The model under review builds one solid part; all positions refer to its coordinate system, in mm. A direction names the side the tool comes from. Round coordinates to 2 decimals unless told otherwise and drop trailing zeros. Write each loop counter-clockwise with the first axis right and the second up, starting at its lowest first coordinate (ties: lowest second). Pieces come first, ordered by that corner, then holes. Notation, with made-up numbers: (8.25, 23) - (20.25, 23) arc R25 cw to (20.25, 35) - close; hole circle Ø4 at (57, 6). An arc over 180 degrees is marked (long way). Return JSON: item names as keys, results as strings.
from build123d import *

# Parameters (mm, degrees)
SKETCH_2_W          = 94.5
SKETCH_2_H          = 98.5
EXTRUDE_1_DEPTH     = 35.7
SHELL_1_T           = -1
SKETCH_5_W          = 35.076830759
SKETCH_5_H          = 6.451639633
CUT_EXTRUDE_1_DEPTH = 2
SKETCH_3_R          = 1.75
CUT_EXTRUDE_2_DEPTH = 2


with BuildPart() as part:
    # 草图2 → 凸台-拉伸1 (new body)
    with BuildSketch(Plane.XY):
        with Locations((47.25, 49.25)):
            Rectangle(SKETCH_2_W, SKETCH_2_H)
    extrude(amount=EXTRUDE_1_DEPTH)

    # 抽壳1
    shell_1_openings = [part.faces().sort_by_distance(p)[0] for p in [
        (47.25, 49.25, 35.7),
    ]]
    offset(amount=SHELL_1_T, openings=shell_1_openings, kind=Kind.INTERSECTION)

    # 草图5 → 切除-拉伸1 (cut, through all)
    with BuildSketch(Plane(origin=(0, 1, 0), x_dir=(1, 0, 0), z_dir=(0, 1, 0))):
        with Locations((47.144981411, -7.555579656)):
            Rectangle(SKETCH_5_W, SKETCH_5_H)
    extrude(amount=-CUT_EXTRUDE_1_DEPTH, mode=Mode.SUBTRACT)

    # 草图3 → 切除-拉伸2 (cut, through all)
    with BuildSketch(Plane.XY.offset(1)):
        with Locations((4.75, 49.25)):
            Circle(SKETCH_3_R)
        with Locations((17.1979618, 19.1979618)):
            Circle(SKETCH_3_R)
        with Locations((47.25, 6.75)):
            Circle(SKETCH_3_R)
        with Locations((77.302038201, 19.1979618)):
            Circle(SKETCH_3_R)
        with Locations((89.75, 49.25)):
            Circle(SKETCH_3_R)
        with Locations((77.302038201, 79.3020382)):
            Circle(SKETCH_3_R)
        with Locations((47.25, 91.75)):
            Circle(SKETCH_3_R)
        with Locations((17.1979618, 79.3020382)):
            Circle(SKETCH_3_R)
    extrude(amount=-CUT_EXTRUDE_2_DEPTH, mode=Mode.SUBTRACT)


solid = part.part
(1) Wall thickness on line 1 (Y direction, x = 47.25, z = 0.7); line 2 (Y direction, x = 58, z = 29); line 3 (X direction, y = 38, z = 26): over which ranges is each line inside the solid? List them lowest first.
Filled in:
{"line 1": "y = 0 to 5, 8.5 to 90, 93.5 to 98.5", "line 2": "y = 0 to 1, 97.5 to 98.5", "line 3": "x = 0 to 1, 93.5 to 94.5"}
(2) Mouldability with a two-part tool opening along Y and no side actions: class faces 3 (the flat face through (47, 98.5, 18)), 4 (the cylindrical face through (48.867, 6.08, 0.507)), 5 (the flat face through (47, 97.5, 18)), 6 (the flat face through (47, 50, 0)) as released by +Y, released by -Y, zero draft, split by the parting line, or undercut.
Filled in:
{"face 3": "released by +Y", "face 4": "undercut", "face 5": "undercut", "face 6": "zero draft"}
(3) Clearance check with flat-ended pins moving along their axes: pin 1 Ø3 at (x, y) = (89.75, 49.25) entering from -Z; pin 2 Ø1.5 at (x, y) = (25.5, 73.5) entering from +Z. State where each tip first meets the part, or that it passes through.
Filled in:
{"pin 1": "passes through", "pin 2": "stops at z = 1"}
(4) For faces 1 (the flat face through (1, 49, 18)), 2 (the cylindrical face through (78.92, 78.63, 0.51)), list the 3-axis set-ups (+Z, -Z, +X, -X, +Y, -Y) from which the entire face can be reached by the end or side of a thin tool; tool diameter is ignored.
Filled in:
{"face 1": "+Z", "face 2": "+Z, -Z"}
(5) Add section C-C (y = 91.75). Write out the cut boundary in (x, z).
Filled in:
{"outline": "(0, 0) - (45.5, 0) - (45.5, 1) - (1, 1) - (1, 35.7) - (0, 35.7) - close; (49, 0) - (94.5, 0) - (94.5, 35.7) - (93.5, 35.7) - (93.5, 1) - (49, 1) - close"}
(6) Add section D-D (z = 16). Write out the cut boundary in (x, y), plus the area to 3 significant figures.
Filled in:
{"outline": "(0, 0) - (94.5, 0) - (94.5, 98.5) - (0, 98.5) - close; hole (1, 1) - (93.5, 1) - (93.5, 97.5) - (1, 97.5) - close", "area": "382 mm2"}
(7) Add section A-A (x = 89.75). Write out the cut boundary in (y, z), plus the area to 3 significant figures.
Filled in:
{"outline": "(0, 0) - (47.5, 0) - (47.5, 1) - (1, 1) - (1, 35.7) - (0, 35.7) - close; (51, 0) - (98.5, 0) - (98.5, 35.7) - (97.5, 35.7) - (97.5, 1) - (51, 1) - close", "area": "164 mm2"}
(8) Add section B-B (y = 49.25). Write out the cut boundary in (x, z), plus the area to 3 significant figures.
Filled in:
{"outline": "(0, 0) - (3, 0) - (3, 1) - (1, 1) - (1, 35.7) - (0, 35.7) - close; (6.5, 0) - (88, 0) - (88, 1) - (6.5, 1) - close; (91.5, 0) - (94.5, 0) - (94.5, 35.7) - (93.5, 35.7) - (93.5, 1) - (91.5, 1) - close", "area": "157 mm2"}
